```python
from build123d import *

# Parameters (mm, degrees)
SKETCH_1_R               = 41.5
SKETCH_1_R_2             = 2
SKETCH_1_R_3             = 10.2
EXTRUDE_1_DEPTH          = 6
CUT_EXTRUDE_1_DEPTH      = 59.99576256
CUT_EXTRUDE_1_DEPTH_BACK = 59.99576256
SKETCH_4_R               = 1.65
SKETCH_3_R               = 25
SKETCH_3_R_2             = 15.9
EXTRUDE_2_DEPTH          = 4
EXTRUDE_START            = -6
SKETCH_5_R               = 43
SKETCH_5_R_2             = 41.5
EXTRUDE_4_DEPTH          = 6


with BuildPart() as part:
    # 草图1 → 凸台-拉伸1 (new body)
    with BuildSketch(Plane.XY):
        Circle(SKETCH_1_R)
        with Locations((0, -37)):
            Circle(SKETCH_1_R_2, mode=Mode.SUBTRACT)
        with Locations((-37, 0)):
            Circle(SKETCH_1_R_2, mode=Mode.SUBTRACT)
        with Locations((0, 37)):
            Circle(SKETCH_1_R_2, mode=Mode.SUBTRACT)
        with Locations((37, 0)):
            Circle(SKETCH_1_R_2, mode=Mode.SUBTRACT)
        Circle(SKETCH_1_R_3, mode=Mode.SUBTRACT)
    extrude(amount=EXTRUDE_1_DEPTH)

    # 草图4 → 切除-拉伸1 (cut, two sides: drawn at the far end of the back side and taken through both)
    with BuildSketch(Plane(origin=(0, 0, 0), x_dir=(-1, 0, 0), z_dir=(0, 0, -1)).offset(-CUT_EXTRUDE_1_DEPTH_BACK)):
        with Locations((-19.798989873, 4.242640687)):
            Circle(SKETCH_4_R)
        with Locations((-4.242640687, 19.798989873)):
            Circle(SKETCH_4_R)
        with Locations((19.798989873, -4.242640687)):
            Circle(SKETCH_4_R)
        with Locations((4.242640687, -19.798989873)):
            Circle(SKETCH_4_R)
    extrude(amount=CUT_EXTRUDE_1_DEPTH + CUT_EXTRUDE_1_DEPTH_BACK, mode=Mode.SUBTRACT)

    # 草图3 → 凸台-拉伸2 (add)
    with BuildSketch(Plane.XY.offset(6)):
        Circle(SKETCH_3_R)
        Circle(SKETCH_3_R_2, mode=Mode.SUBTRACT)
    extrude(amount=EXTRUDE_2_DEPTH)

    # 草图5 → 凸台-拉伸4 (add)
    with BuildSketch(Plane.XY.offset(6).offset(EXTRUDE_START)):
        Circle(SKETCH_5_R)
        Circle(SKETCH_5_R_2, mode=Mode.SUBTRACT)
    extrude(amount=EXTRUDE_4_DEPTH)


solid = part.part
```
The listing builds one solid part. Answer for the finished solid, in the listing's coordinates (mm). A direction names the side the tool comes from. Coordinates: 2 decimals unless noted, no trailing zeros. Loops run counter-clockwise (first coordinate to the right, second up) from the corner with the lowest first, then second, coordinate; pieces in that order, holes last. Notation, with made-up numbers: (57, -11.5) - (71, -11.5) arc R22 cw to (71, 4.5) - close; hole circle Ø6 at (41, -24). An arc over 180 degrees is marked (long way). Write item = value, one per line.
1) Find the intervals of material crossed by line 1 along Y through (x, z) = (0, 1.85); line 2 along X through (y, z) = (4, 0.75); line 3 along Z through (x, y) = (36.5, 22), in increasing order.
Responses:
line_1 = -43 to -39, -35 to -10.2, 10.2 to 35, 39 to 43
line_2 = -42.81 to -9.38, 9.38 to 18.17, 21.43 to 42.81
line_3 = 0 to 6
2) Section D-D (x = 12) is taken. Determine the outline of the cut face in (y, z).
Responses:
outline = (-41.29, 0) - (41.29, 0) - (41.29, 6) - (21.93, 6) - (21.93, 10) - (10.43, 10) - (10.43, 6) - (-10.43, 6) - (-10.43, 10) - (-21.93, 10) - (-21.93, 6) - (-41.29, 6) - close
3) Section A-A (x = 0) is taken. Determine the outline of the cut face in (y, z), plus the area to 3 significant figures.
Responses:
outline = (-43, 0) - (-39, 0) - (-39, 6) - (-43, 6) - close; (-35, 0) - (-10.2, 0) - (-10.2, 6) - (-15.9, 6) - (-15.9, 10) - (-25, 10) - (-25, 6) - (-35, 6) - close; (10.2, 0) - (35, 0) - (35, 6) - (25, 6) - (25, 10) - (15.9, 10) - (15.9, 6) - (10.2, 6) - close; (39, 0) - (43, 0) - (43, 6) - (39, 6) - close
area = 418 mm^2
4) Determine the mould class of faces 1 (the face through (4.707, -9.049, 2.958)), 2 (the face through (-5.598, 42.634, 2.958)), 3 (the face through (9, -9, 0)) for opening direction X: pulls with the +X half, pulls with the -X half, needs draft (parallel to the pull), parting line crosses it, or undercut.
Responses:
face_1 = undercut
face_2 = parting line crosses it
face_3 = needs draft
5) Each of these flat-tipped pins is pushed along its axis until it touches: P1, Ø5.5, axis at x = 4.24, y = 19.8, coming from the -Z side; P2, Ø4, axis at x = -3.5, y = -31.5, coming from the +Z side; P3, Ø2, axis at x = -4.24, y = -19.8, coming from the -Z side; P4, Ø6, axis at y = -32.5, z = 6.5, coming from the +X side. Where does it stop, or does it pass through?
Responses:
P1 = 0
P2 = 6
P3 = 6
P4 = 31.25
6) Which of the six approach directions +Z, -Z, +X, -X, +Y, -Y give full straight-line access (tool end or side, diameter ignored) to faces 4 (the face through (19, -19, 6)), 5 (the face through (21.11, 3.24, 3.04)), 6 (the face through (-0.3, -16.3, 10))?
Responses:
face_4 = +Z
face_5 = -Z
face_6 = +Z, +X, -X, +Y, -Y
7) Section C-C (y = -9) is taken. Determine the outline of the cut face in (x, z).
Responses:
outline = (-42.05, 0) - (-4.8, 0) - (-4.8, 6) - (-13.11, 6) - (-13.11, 10) - (-23.32, 10) - (-23.32, 6) - (-42.05, 6) - close; (4.8, 0) - (42.05, 0) - (42.05, 6) - (23.32, 6) - (23.32, 10) - (13.11, 10) - (13.11, 6) - (4.8, 6) - close
